Part model, mm, in its own coordinate system. Coordinates: 2 decimals unless noted, no trailing zeros. Loops run counter-clockwise (first coordinate to the right, second up) from the corner with the lowest first, then second, coordinate; pieces in that order, holes last. Notation, with made-up numbers: M -5.5,-22 L 36.5,-22 A19 cw 36.5,-13 Z; hole C 57,11 d3. An arc over 180 degrees is marked long. Answer as CSV lines item,"result". Start each with the question number.
from build123d import *

# Parameters (mm, degrees)
SKETCH1_R                               = 31.5
ELBOW_PLATE_DEPTH                       = 4
SKETCH3_R                               = 1.33
SCREW_HOLES_DEPTH                       = 45.726949371
CABLE_SLOT_DEPTH                        = 4
FILLET1_R                               = 2
CBORE_FOR_M6_HEX_HEAD_BOLT1_D           = 2
CBORE_FOR_M6_HEX_HEAD_BOLT1_CBORE_D     = 3.5
CBORE_FOR_M6_HEX_HEAD_BOLT1_CBORE_DEPTH = 1


with BuildPart() as part:
    # Sketch1 → Elbow Plate (new body)
    with BuildSketch(Plane.XY):
        Circle(SKETCH1_R)
    extrude(amount=ELBOW_PLATE_DEPTH)

    # Sketch3 → Screw Holes (cut, through all)
    with BuildSketch(Plane(origin=(0, 0, 0), x_dir=(-1, 0, 0), z_dir=(0, 0, -1))):
        with Locations((22.9496732, 13.25)):
            Circle(SKETCH3_R)
        with Locations((0, 26.5)):
            Circle(SKETCH3_R)
        with Locations((22.9496732, -13.25)):
            Circle(SKETCH3_R)
        with Locations((0, -26.5)):
            Circle(SKETCH3_R)
        with Locations((-22.9496732, -13.25)):
            Circle(SKETCH3_R)
        with Locations((-22.9496732, 13.25)):
            Circle(SKETCH3_R)
    extrude(amount=-SCREW_HOLES_DEPTH, mode=Mode.SUBTRACT)

    # Sketch4 → Cable Slot (cut)
    with BuildSketch(Plane.XY.offset(4)):
        with BuildLine():
            ThreePointArc((0, -23.172318516), (4.086159258, -19.086159258), (0, -15))
            ThreePointArc((0, -15), (-15, 0), (0, 15))
            ThreePointArc((0, 15), (4.086159258, 19.086159258), (0, 23.172318516))
            ThreePointArc((0, 23.172318516), (-23.172318516, 0), (0, -23.172318516))
        make_face()
    extrude(amount=-CABLE_SLOT_DEPTH, mode=Mode.SUBTRACT)

    # Fillet1
    fillet1_edges = [part.edges().sort_by_distance(p)[0] for p in [
        (-23.172318516, 0, 0),
        (4.086159258, 19.086159258, 0),
        (-15, 0, 0),
        (4.086159258, -19.086159258, 0),
    ]]
    fillet(fillet1_edges, radius=FILLET1_R)

    # CBORE for M6 Hex Head Bolt1 (through all)
    with Locations(Plane(origin=(12, 0, 0), x_dir=(-1, 0, 0), z_dir=(0, 0, -1))):
        with Locations((0, 0), (3.514718626, 8.485281374), (12, 12), (20.485281374, 8.485281374), (24, 0), (20.485281374, -8.485281374), (12, -12), (3.514718626, -8.485281374)):
            CounterBoreHole(CBORE_FOR_M6_HEX_HEAD_BOLT1_D / 2, CBORE_FOR_M6_HEX_HEAD_BOLT1_CBORE_D / 2, CBORE_FOR_M6_HEX_HEAD_BOLT1_CBORE_DEPTH)


solid = part.part
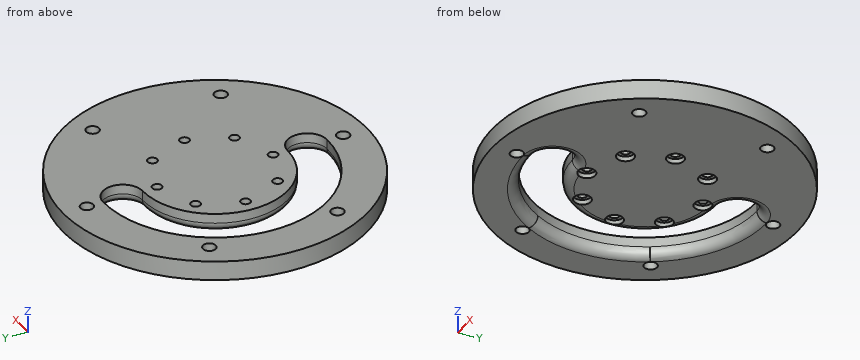
Q1. Flat gauge pins, fed straight in: P1, Ø1, axis at x = 8, y = -9, coming from the -Z side; P2, Ø2, axis at y = -8.5, z = 1, coming from the +X side; P3, Ø1.5, axis at y = 17, z = 0.5, coming from the +X side. Where does each tip first touch, or does it go through?
Q2. Wall check: L1, parallel to Y at x = -9, z = 1.65; L2, parallel to Y at x = -2.5, z = 1.95; L3, parallel to X at y = -11.5, z = 3.7. Give the ranges that are in metal, low to high.
Q3. Slice it at A-A, the plane x = 23. Write the cut outline in (y, z), and give its area (3 significant figures).
Q4. Slice it at D-D, the plane y = 0. Write the cut outline in (x, z).
Q5. Slice it at C-C, the plane z = 3.35. State how many separate pieces and enclosed holes the cut face has, and give its area (3 significant figures).
Q6. Slice it at B-B, the plane y = 26.5. Write the cut outline in (x, z), and give its area (3 significant figures).
Solved:
1,P1,"stops at z = 1"
1,P2,"stops at x = 30.59"
1,P3,"stops at x = 26.98"
2,L1,"y = -30.19 to -21.39, -11.96 to -9.34, -7.63 to 7.63, 9.34 to 11.96, 21.39 to 30.19"
2,L2,"y = -31.4 to -23.04, -14.79 to 14.79, 23.04 to 31.4"
2,L3,"x = -29.33 to -20.12, -9.63 to -0.87, 0.87 to 29.33"
3,outline,"M -21.52,0 L -14.58,0 L -14.58,4 L -21.52,4 Z; M -11.92,0 L 11.92,0 L 11.92,4 L -11.92,4 Z; M 14.58,0 L 21.52,0 L 21.52,4 L 14.58,4 Z"
3,area,"151 mm2"
4,outline,"M -31.5,0 L -25.17,0 A2 ccw -23.17,2 L -23.17,4 L -31.5,4 Z; M -15,2 A2 ccw -13.75,0.15 L -13.75,1 L -13,1 L -13,4 L -15,4 Z; M -11,1 L -10.25,1 L -10.25,0 L 10.25,0 L 10.25,1 L 11,1 L 11,4 L -11,4 Z; M 13,1 L 13.75,1 L 13.75,0 L 31.5,0 L 31.5,4 L 13,4 Z"
5,separate pieces,"1"
5,enclosed holes,"15"
5,area,"2,520 mm2"
6,outline,"M -17.03,0 L -1.33,0 L -1.33,4 L -17.03,4 Z; M 1.33,0 L 17.03,0 L 17.03,4 L 1.33,4 Z"
6,area,"126 mm2"
